from build123d import *

# Parameters (mm, degrees)
BOSS_EXTRUDE1_DEPTH = 2
SKETCH2_R           = 3
SKETCH2_R_2         = 2.5
BOSS_EXTRUDE2_DEPTH = 3
SKETCH3_R           = 1
CUT_EXTRUDE1_DEPTH  = 1
SKETCH4_R           = 0.5
CUT_EXTRUDE2_DEPTH  = 1


with BuildPart() as part:
    # Sketch1 → Boss-Extrude1 (new body)
    with BuildSketch(Plane.XY):
        with BuildLine():
            Line((1.2, -6.33), (1.8, -4.1378116))
            ThreePointArc((1.8, -4.1378116), (2.058560194, -3.569045514), (2.48, -3.1078116))
            ThreePointArc((2.48, -3.1078116), (2.641475661, -2.955390865), (2.794244497, -2.794244497))
            ThreePointArc((2.794244497, -2.794244497), (2.955390865, -2.641475661), (3.1078116, -2.48))
            ThreePointArc((3.1078116, -2.48), (3.569045514, -2.058560194), (4.1378116, -1.8))
            Line((4.1378116, -1.8), (6.33, -1.2))
            ThreePointArc((6.33, -1.2), (6.992020752, -0.754882576), (7.25, 0))
            ThreePointArc((7.25, 0), (6.992020752, 0.754882576), (6.33, 1.2))
            Line((6.33, 1.2), (4.1378116, 1.8))
            ThreePointArc((4.1378116, 1.8), (3.569045514, 2.058560194), (3.1078116, 2.48))
            ThreePointArc((3.1078116, 2.48), (2.955390865, 2.641475661), (2.794244497, 2.794244497))
            ThreePointArc((2.794244497, 2.794244497), (2.641475661, 2.955390865), (2.48, 3.1078116))
            ThreePointArc((2.48, 3.1078116), (2.058560194, 3.569045514), (1.8, 4.1378116))
            Line((1.8, 4.1378116), (1.2, 6.33))
            ThreePointArc((1.2, 6.33), (0.754882576, 6.992020752), (0, 7.25))
            ThreePointArc((0, 7.25), (-0.754882576, 6.992020752), (-1.2, 6.33))
            Line((-1.2, 6.33), (-1.8, 4.1378116))
            ThreePointArc((-1.8, 4.1378116), (-2.058560194, 3.569045514), (-2.48, 3.1078116))
            ThreePointArc((-2.48, 3.1078116), (-2.641475661, 2.955390865), (-2.794244497, 2.794244497))
            ThreePointArc((-2.794244497, 2.794244497), (-2.955390865, 2.641475661), (-3.1078116, 2.48))
            ThreePointArc((-3.1078116, 2.48), (-3.569045514, 2.058560194), (-4.1378116, 1.8))
            Line((-4.1378116, 1.8), (-6.33, 1.2))
            ThreePointArc((-6.33, 1.2), (-6.992020752, 0.754882576), (-7.25, 0))
            ThreePointArc((-7.25, 0), (-6.992020752, -0.754882576), (-6.33, -1.2))
            Line((-6.33, -1.2), (-4.1378116, -1.8))
            ThreePointArc((-4.1378116, -1.8), (-3.569045514, -2.058560194), (-3.1078116, -2.48))
            ThreePointArc((-3.1078116, -2.48), (-2.955390865, -2.641475661), (-2.794244497, -2.794244497))
            ThreePointArc((-2.794244497, -2.794244497), (-2.641475661, -2.955390865), (-2.48, -3.1078116))
            ThreePointArc((-2.48, -3.1078116), (-2.058560194, -3.569045514), (-1.8, -4.1378116))
            Line((-1.8, -4.1378116), (-1.2, -6.33))
            ThreePointArc((-1.2, -6.33), (-0.754882576, -6.992020752), (0, -7.25))
            ThreePointArc((0, -7.25), (0.754882576, -6.992020752), (1.2, -6.33))
        make_face()
    extrude(amount=BOSS_EXTRUDE1_DEPTH)

    # Sketch2 → Boss-Extrude2 (add)
    with BuildSketch(Plane(origin=(0, 0, 0), x_dir=(-1, 0, 0), z_dir=(0, 0, -1))):
        Circle(SKETCH2_R)
        Circle(SKETCH2_R_2, mode=Mode.SUBTRACT)
    extrude(amount=BOSS_EXTRUDE2_DEPTH)

    # Sketch3 → Cut-Extrude1 (cut)
    with BuildSketch(Plane.XY.offset(2)):
        Circle(SKETCH3_R)
    extrude(amount=-CUT_EXTRUDE1_DEPTH, mode=Mode.SUBTRACT)

    # Sketch4 → Cut-Extrude2 (cut)
    with BuildSketch(Plane.XY.offset(1)):
        Circle(SKETCH4_R)
    extrude(amount=-CUT_EXTRUDE2_DEPTH, mode=Mode.SUBTRACT)


solid = part.part
Model file for the job. Use its own axes, mm. A direction names the side the tool comes from. Give positions to 0.01 mm unless a question says otherwise; leave off trailing zeros. Loops run counter-clockwise (first coordinate to the right, second up) from the corner with the lowest first, then second, coordinate; pieces in that order, holes last.
1) Saw through at C-C (y = -6). Write the cut outline in (x, z), plus the area to 3 significant figures.
2) Saw through at D-D (z = -2.2). Write the cut outline in (x, y).
3) Saw through at B-B (x = 6.75). Write the cut outline in (y, z), plus the area to 3 significant figures.
4) Pull direction Y, two halves, no side cores. Call faces 1 (the flat face through (5.219, -1.504, 0.986)), 2 (the cylindrical face through (0.54, -2.44, -1.48)), 3 (the flat face through (0, -2, 2)): +Y half, -Y half, draft (parallel to the pull), parting line (faces both ways), or undercut.
5) Tool access for faces 4 (the cylindrical face through (-0.108, -0.488, 0.507)), 5 (the flat face through (1, 0, 0)): list every direction of +Z, -Z, +X, -X, +Y, -Y with a clear straight run to the whole face (end or side of a thin tool).
6) Flat gauge pins, fed straight in: pin 1 Ø1 at (x, z) = (-1, -2) entering from -Y; pin 2 Ø2.5 at (x, y) = (-0.5, 0) entering from -Z. Where does each tip first touch, or does it go through?
7) Wall check: line 1 (Y direction, x = 0, z = -0.7); line 2 (X direction, y = 0.75, z = 1.65); line 3 (Y direction, x = 0.75, z = -1.45). Give the ranges that are in metal, low to high.
Answer block:
1. outline: (-1.29, 0) - (1.29, 0) - (1.29, 2) - (-1.29, 2) - close
1. area: 5.16 mm2
2. outline: circle Ø6 at (0, 0); hole circle Ø5 at (0, 0)
3. outline: (-0.99, 0) - (0.99, 0) - (0.99, 2) - (-0.99, 2) - close
3. area: 3.98 mm2
4. face 1: -Y half
4. face 2: undercut
4. face 3: draft
5. face 4: +Z, -Z
5. face 5: -Z
6. pin 1: stops at y = -2.96
6. pin 2: stops at z = 0
7. line 1: y = -3 to -2.5, 2.5 to 3
7. line 2: x = -7 to -0.66, 0.66 to 7
7. line 3: y = -2.9 to -2.38, 2.38 to 2.9
